For this review, take the finished solid that the model builds, in its own axes (mm). Face numbers are marked on the shaded views. A direction names the side the tool comes from. Coordinates: 2 decimals unless noted, no trailing zeros. Write each loop counter-clockwise with the first axis right and the second up, starting at its lowest first coordinate (ties: lowest second). Pieces come first, ordered by that corner, then holes.
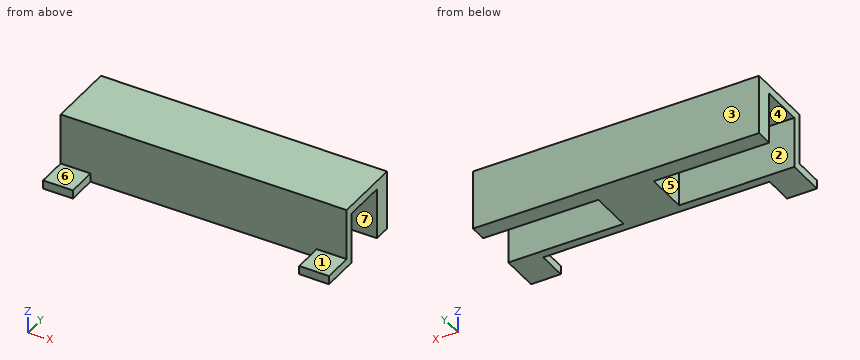
```python
from build123d import *

# Parameters (mm, degrees)
BOX003_W     = 7
BOX003_H     = 9
BOX003_DEPTH = 2
BOX004_W     = 7
BOX004_H     = 9
BOX004_DEPTH = 2
BOX002_W     = 27
BOX002_H     = 10
BOX002_DEPTH = 12
BOX001_W     = 27
BOX001_H     = 10
BOX001_DEPTH = 12
BOX_W        = 67
BOX_H        = 16
BOX_DEPTH    = 14


with BuildPart() as cubo003:
    # Box003 → Box003 (new body)
    with BuildSketch(Plane(origin=(0, -7, 0), x_dir=(1, 0, 0), z_dir=(0, 0, 1))):
        with Locations((3.5, 4.5)):
            Rectangle(BOX003_W, BOX003_H)
    extrude(amount=BOX003_DEPTH)


with BuildPart() as fusion:
    # Box004 → Box004 (new body)
    with BuildSketch(Plane(origin=(60, -7, 0), x_dir=(1, 0, 0), z_dir=(0, 0, 1))):
        with Locations((3.5, 4.5)):
            Rectangle(BOX004_W, BOX004_H)
    extrude(amount=BOX004_DEPTH)

    # Fusion: union Cubo003
    add(cubo003.part)


with BuildPart() as cubo002:
    # Box002 → Box002 (new body)
    with BuildSketch(Plane(origin=(40, 2, 0), x_dir=(1, 0, 0), z_dir=(0, 0, 1))):
        with Locations((13.5, 5)):
            Rectangle(BOX002_W, BOX002_H)
    extrude(amount=BOX002_DEPTH)


with BuildPart() as cubo001:
    # Box001 → Box001 (new body)
    with BuildSketch(Plane(origin=(0, 2, 0), x_dir=(1, 0, 0), z_dir=(0, 0, 1))):
        with Locations((13.5, 5)):
            Rectangle(BOX001_W, BOX001_H)
    extrude(amount=BOX001_DEPTH)


with BuildPart() as fusion001:
    # Box → Box (new body)
    with BuildSketch(Plane.XY):
        with Locations((33.5, 8)):
            Rectangle(BOX_W, BOX_H)
    extrude(amount=BOX_DEPTH)

    # Cut: cut Cubo001
    add(cubo001.part, mode=Mode.SUBTRACT)

    # Cut001: cut Cubo002
    add(cubo002.part, mode=Mode.SUBTRACT)

    # Fusion001: union Fusion
    add(fusion.part)


solid = fusion001.part
```
Q1. Add section D-D (z = 3.75). State the section outline as (x, y) points, then the cut area to 3 significant figures.
Ans:
outline: (0, 0) - (67, 0) - (67, 2) - (40, 2) - (40, 12) - (67, 12) - (67, 16) - (0, 16) - (0, 12) - (27, 12) - (27, 2) - (0, 2) - close
area: 532 mm2
Q2. Clearance check with flat-ended pins moving along their axes: pin 1 Ø2 at (x, y) = (54, 7) entering from -Z; pin 2 Ø7 at (x, z) = (22.5, 6) entering from -Y; pin 3 Ø5.5 at (x, y) = (65, -4) entering from +Z. State where each tip first meets the part, or that it passes through.
Ans:
pin 1: stops at z = 12
pin 2: stops at y = 0
pin 3: stops at z = 2
Q3. Add section C-C (y = 11). State the section outline as (x, z) points, then the cut area to 3 significant figures.
Ans:
outline: (0, 12) - (27, 12) - (27, 0) - (40, 0) - (40, 12) - (67, 12) - (67, 14) - (0, 14) - close
area: 290 mm2
Q4. Draft analysis for pull direction Y (two halves, no side actions). For the marked faces 1, 2, 3 and 4, state which applies: +Y half, -Y half, draft (parallel to the pull), parting line (faces both ways), or undercut.
Ans:
face 1: draft
face 2: undercut
face 3: +Y half
face 4: undercut
Q5. Add section B-B (x = 4). State the section outline as (y, z) points.
Ans:
outline: (-7, 0) - (2, 0) - (2, 12) - (12, 12) - (12, 0) - (16, 0) - (16, 14) - (0, 14) - (0, 2) - (-7, 2) - close
Q6. Tool access review of the marked faces 5, 6 and 7: name each direction out of +Z, -Z, +X, -X, +Y, -Y from which nothing blocks a thin tool from reaching the whole face with its end or side.
Ans:
face 5: -Z, -X
face 6: +Z, +X, -X, -Y
face 7: -Z, +X
Q7. Add section A-A (y = -2). State the section outline as (x, z) points.
Ans:
outline: (0, 0) - (7, 0) - (7, 2) - (0, 2) - close; (60, 0) - (67, 0) - (67, 2) - (60, 2) - close
Q8. For probe 1 along Y at (x, z) = (24.5, 3); probe 2 along Y at (x, z) = (32.5, 1.5); probe 3 along Z at (x, y) = (24.5, 5.25), list the stretches that pass through material, from the lowest coordinate up.
Ans:
probe 1: y = 0 to 2, 12 to 16
probe 2: y = 0 to 16
probe 3: z = 12 to 14
